```python
from build123d import *

# Parameters (mm, degrees)
BOSS_EXTRUDE1_START = -10.05
BOSS_EXTRUDE1_DEPTH = 20.1
CUT_EXTRUDE1_DEPTH  = 30.8
SKETCH5_R           = 5
BOSS_EXTRUDE2_DEPTH = 1.3
SKETCH6_R           = 2.4
BOSS_EXTRUDE3_DEPTH = 4
SKETCH8_W           = 7
SKETCH8_H           = 3
BOSS_EXTRUDE4_DEPTH = 5


with BuildPart() as part:
    # Sketch3 → Boss-Extrude1 (new body)
    with BuildSketch(Plane.XY.offset(BOSS_EXTRUDE1_START)):
        Polygon((-30.75, 0), (-30.75, 26.8), (-37.5, 26.8), (-37.5, 29.8), (-30.75, 29.8), (-30.75, 37.5), (10.05, 37.5), (10.05, 29.8), (16.8, 29.8), (16.8, 26.8), (10.05, 26.8), (10.05, 0), align=None)
    extrude(amount=BOSS_EXTRUDE1_DEPTH)

    # Sketch4 → Cut-Extrude1 (cut, through all)
    with BuildSketch(Plane(origin=(0, 29.8, 0), x_dir=(1, 0, 0), z_dir=(0, 1, 0))):
        with BuildLine():
            Line((-37.5, 6), (-37.5, 4))
            Line((-37.5, 4), (-36.332050808, 4))
            ThreePointArc((-36.332050808, 4), (-32.6, 5), (-36.332050808, 6))
            Line((-36.332050808, 6), (-37.5, 6))
        make_face()
        with BuildLine():
            Line((16.8, -6), (15.632050808, -6))
            ThreePointArc((15.632050808, -6), (11.9, -5), (15.632050808, -4))
            Line((15.632050808, -4), (16.8, -4))
            Line((16.8, -4), (16.8, -6))
        make_face()
        with BuildLine():
            Line((-37.5, -4), (-37.5, -6))
            Line((-37.5, -6), (-36.332050808, -6))
            ThreePointArc((-36.332050808, -6), (-32.6, -5), (-36.332050808, -4))
            Line((-36.332050808, -4), (-37.5, -4))
        make_face()
        with BuildLine():
            Line((16.8, 4), (15.632050808, 4))
            ThreePointArc((15.632050808, 4), (11.9, 5), (15.632050808, 6))
            Line((15.632050808, 6), (16.8, 6))
            Line((16.8, 6), (16.8, 4))
        make_face()
    extrude(amount=-CUT_EXTRUDE1_DEPTH, mode=Mode.SUBTRACT)

    # Sketch5 → Boss-Extrude2 (add)
    with BuildSketch(Plane(origin=(0, 37.5, 0), x_dir=(1, 0, 0), z_dir=(0, 1, 0))):
        Circle(SKETCH5_R)
    extrude(amount=BOSS_EXTRUDE2_DEPTH)

    # Sketch6 → Boss-Extrude3 (add)
    with BuildSketch(Plane(origin=(0, 38.8, 0), x_dir=(1, 0, 0), z_dir=(0, 1, 0))):
        Circle(SKETCH6_R)
    extrude(amount=BOSS_EXTRUDE3_DEPTH)

    # Sketch8 → Boss-Extrude4 (add)
    with BuildSketch(Plane(origin=(10.05, 0, 0), x_dir=(0, 0, -1), z_dir=(1, 0, 0))):
        with Locations((0, 5.5)):
            Rectangle(SKETCH8_W, SKETCH8_H)
    extrude(amount=BOSS_EXTRUDE4_DEPTH)


solid = part.part
```
CAD build for the part. Positions are in the model's coordinates, mm. A direction names the side the tool comes from. Coordinates: 2 decimals unless noted, no trailing zeros. Order: outer loops, then holes, each group sorted by start corner. A loop starts at its lowest first (then second) coordinate and runs counter-clockwise, first axis right, second up. Notation, with made-up numbers: M -20,11 L 34,11 A18 cw 34,21 Z; hole C 58.25,5 d9. An arc over 180 degrees is marked long. Answer as CSV lines item,"result".
1) Mould opens along Z. For faces 5 (the flat face through (-30.75, 13, 0)), 6 (the flat face through (16, 28, -4)), 7 (the flat face through (-10, 19, -10.05)) say: released by +Z, released by -Z, zero draft, split by the parting line, or undercut.
Verdict:
face 5,"zero draft"
face 6,"undercut"
face 7,"released by -Z"
2) Drill centre lines: L1, parallel to Y at x = -29, z = 7.25; L2, parallel to X at y = 14, z = -0.5; L3, parallel to Y at x = -31, z = -7.5. Where is each one in solid material? Low to high. Write a range as from..to.
Verdict:
L1,"0..37.5"
L2,"-30.75..10.05"
L3,"26.8..29.8"
3) Cut at C-C (x = 0). List the corners of the cut face in (y, z).
Verdict:
outline,"M 0,-10.05 L 37.5,-10.05 L 37.5,-5 L 38.8,-5 L 38.8,-2.4 L 42.8,-2.4 L 42.8,2.4 L 38.8,2.4 L 38.8,5 L 37.5,5 L 37.5,10.05 L 0,10.05 Z"
4) Flat gauge pins, fed straight in: P1, Ø2.5, axis at x = 11.5, y = 5.5, coming from the -Z side; P2, Ø2.5, axis at y = 33, z = 1.5, coming from the -X side; P3, Ø1, axis at x = -20, z = -4, coming from the +Y side; P4, Ø2.5, axis at x = -34.6, z = -5, coming from the -Y side. Where does each tip first touch, or does it go through?
Verdict:
P1,"z = -3.5"
P2,"x = -30.75"
P3,"y = 37.5"
P4,"through"
5) 3-axis set-ups, long thin cutter, end or side, ignore diameter. For faces 1 (the cylindrical face through (11.9, 28.32, 5.07)), 2 (the flat face through (-37, 28, -6)), 3 (the flat face through (-34, 29.8, 0)), 4 (the flat face through (13, 29.8, 0)): which of +Z, -Z, +X, -X, +Y, -Y reach the whole face in a straight line?
Verdict:
face 1,"+Y"
face 2,"-X, +Y, -Y"
face 3,"+Z, -Z, -X, +Y"
face 4,"+Z, -Z, +X, +Y"
6) Cut at B-B (z = -9). List the corners of the cut face in (x, y), then the cut area to 3 significant figures.
Verdict:
outline,"M -37.5,26.8 L -30.75,26.8 L -30.75,0 L 10.05,0 L 10.05,26.8 L 16.8,26.8 L 16.8,29.8 L 10.05,29.8 L 10.05,37.5 L -30.75,37.5 L -30.75,29.8 L -37.5,29.8 Z"
area,"1,570 mm2"
7) Cut at A-A (x = 11). List the corners of the cut face in (y, z).
Verdict:
outline,"M 4,-3.5 L 7,-3.5 L 7,3.5 L 4,3.5 Z; M 26.8,-10.05 L 29.8,-10.05 L 29.8,10.05 L 26.8,10.05 Z"
8) Cut at D-D (y = 21.5). List the corners of the cut face in (x, z).
Verdict:
outline,"M -30.75,-10.05 L 10.05,-10.05 L 10.05,10.05 L -30.75,10.05 Z"
